Design review of the part shown in the three views and the two pictorial views. Dimensions are in mm from the part's minimum x, y and z. Round coordinates to 2 decimals unless told otherwise and drop trailing zeros. Order: outer loops, then holes, each group sorted by start corner. A loop starts at its lowest first (then second) coordinate and runs counter-clockwise, first axis right, second up.
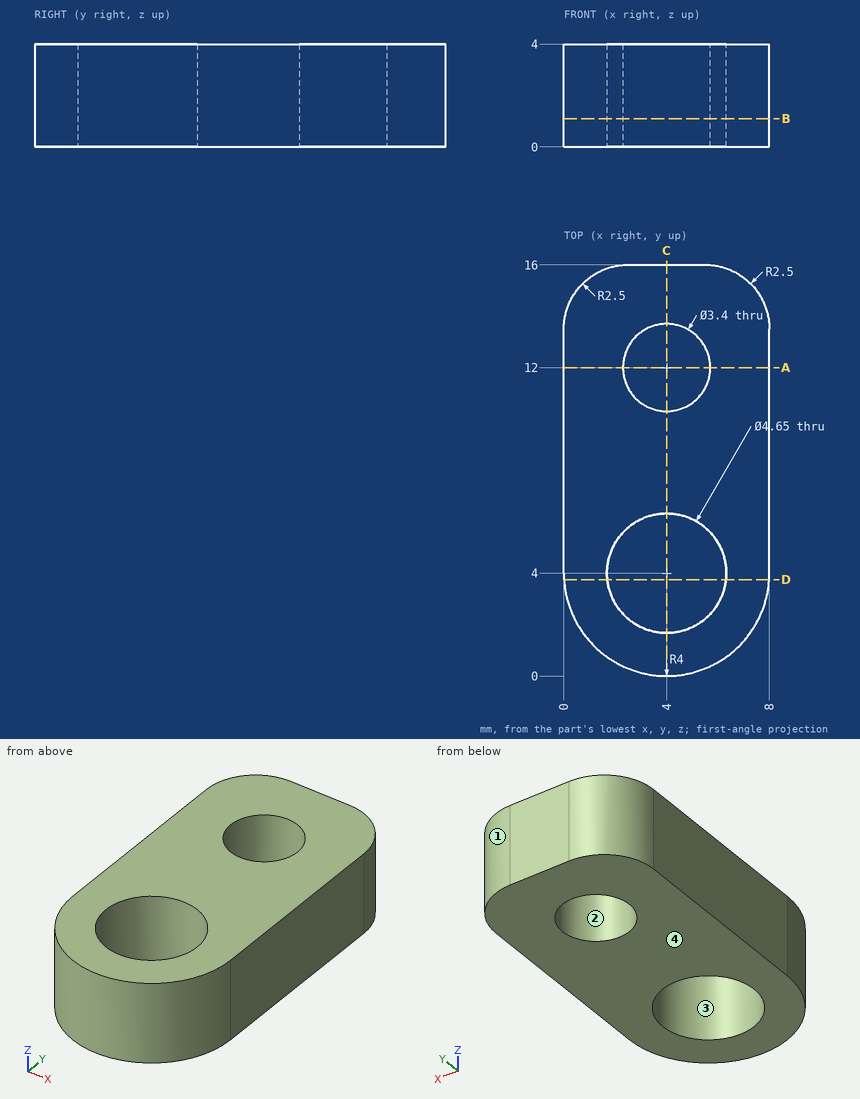
1) Take a section at A-A on y = 12. Give the boundary of the cut face in (x, z).
Results:
outline: (0, 0) - (2.3, 0) - (2.3, 4) - (0, 4) - close; (5.7, 0) - (8, 0) - (8, 4) - (5.7, 4) - close
2) The part is to be moulded in two halves that separate along X. For the marked faces 1, 2, 3 and 4, say which applies: released by +X, released by -X, zero draft, split by the parting line, or undercut.
Results:
face 1: released by +X
face 2: undercut
face 3: undercut
face 4: zero draft
3) To check wall thickness, follow line 1 along Y through (x, z) = (4, 1.45) (3 decimals); line 2 along Y through (x, z) = (5.25, 1); line 3 along X through (y, z) = (4, 2.75) (3 decimals). State the ranges of each line that lie inside material, in increasing order.
Results:
line 1: y = 0 to 1.675, 6.325 to 10.3, 13.7 to 16
line 2: y = 0.2 to 2.04, 5.96 to 10.85, 13.15 to 16
line 3: x = 0 to 1.675, 6.325 to 8
4) Take a section at B-B on z = 1.1. Give the boundary of the cut face in (x, y) (3 decimals), plus the area to 3 significant figures.
Results:
outline: (0, 4) arc R4 ccw to (8, 4) - (8, 13.5) arc R2.5 ccw to (5.5, 16) - (2.5, 16) arc R2.5 ccw to (0, 13.5) - close; hole circle Ø4.65 at (4, 4); hole circle Ø3.4 at (4, 12)
area: 92.4 mm2
5) Take a section at C-C on x = 4. Give the boundary of the cut face in (y, z) (3 decimals), plus the area to 3 significant figures.
Results:
outline: (0, 0) - (1.675, 0) - (1.675, 4) - (0, 4) - close; (6.325, 0) - (10.3, 0) - (10.3, 4) - (6.325, 4) - close; (13.7, 0) - (16, 0) - (16, 4) - (13.7, 4) - close
area: 31.8 mm2
6) Take a section at D-D on y = 3.75. Give the boundary of the cut face in (x, z), plus the area to 3 significant figures.
Results:
outline: (0.01, 0) - (1.69, 0) - (1.69, 4) - (0.01, 4) - close; (6.31, 0) - (7.99, 0) - (7.99, 4) - (6.31, 4) - close
area: 13.4 mm2
